Check sheet for the drawn part. Datum: minimum x, y, z corner. Units: mm. A direction names the side the tool comes from. Round coordinates to 2 decimals unless told otherwise and drop trailing zeros. Order: outer loops, then holes, each group sorted by start corner. A loop starts at its lowest first (then second) coordinate and runs counter-clockwise, first axis right, second up. Notation, with made-up numbers: (-15.75, 7) -> (41.25, 7) arc R13 cw to (41.25, 26) -> close; hole circle Ø7 at (-29.75, 34.25). An arc over 180 degrees is marked (long way). Answer as a JSON object with one key per item and string values. Group by question number.
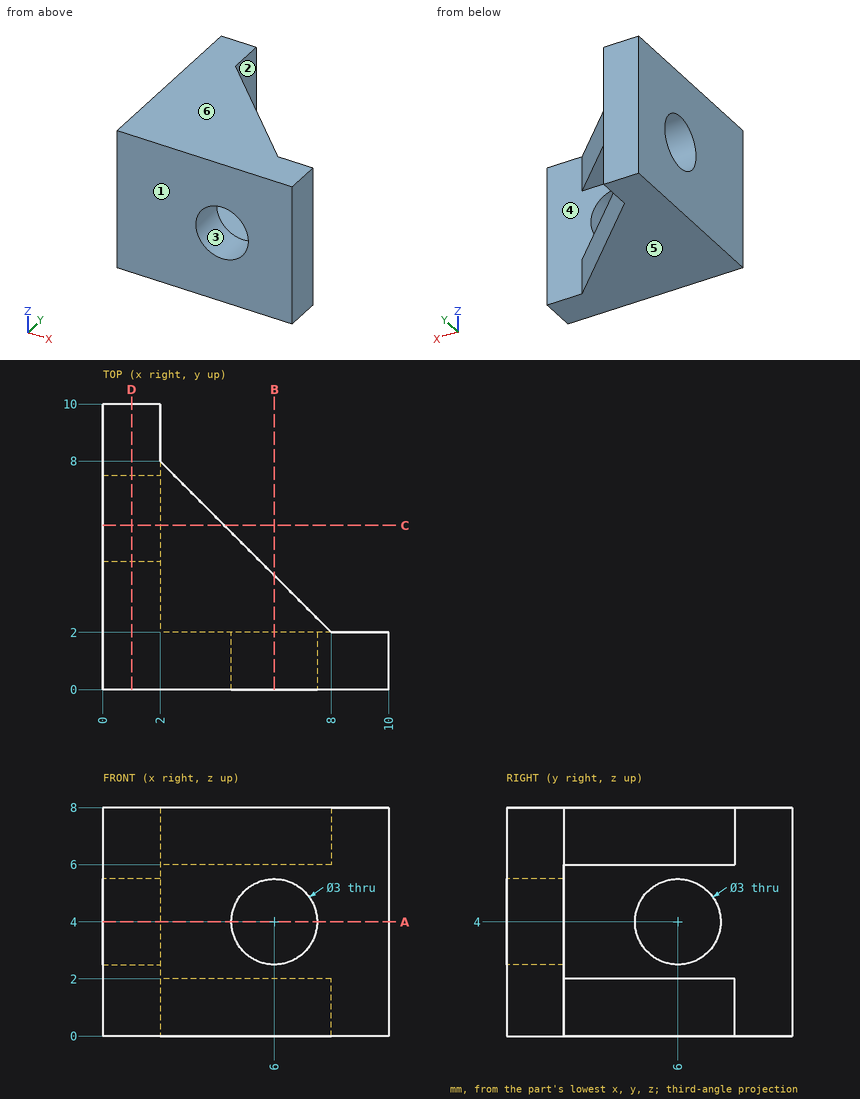
Item 1: Thickness scan on L1, parallel to Z at x = 6, y = 0.5; L2, parallel to Y at x = 0.8, z = 4; L3, parallel to Z at x = 4, y = 2.5. Record the ranges inside material, lowest first.
Item 2: Sectioned sample at D-D, the plane x = 1. Enter the section's corners in (y, z).
Item 3: Sectioned sample at A-A, the plane z = 4. Enter the section's corners in (x, y), then the cut area to 3 significant figures.
Item 4: Mould release check, pull along Z, two halves, no side actions. Record for the marked faces 3, 4, 5 and 6: pulls with the +Z half, pulls with the -Z half, needs draft (parallel to the pull), parting line crosses it, or undercut.
Item 5: Set-up check for the marked faces 1 and 2: record each of +Z, -Z, +X, -X, +Y, -Y from which the full face is reachable in a straight line by a thin tool's end or side.
Item 6: Sectioned sample at B-B, the plane x = 6. Enter the section's corners in (y, z).
Item 7: Depth check by flat-ended pin: pin 1 Ø1 at (y, z) = (3, 2) entering from +X; pin 2 Ø3 at (y, z) = (8.5, 2.5) entering from +X. Enter the tip coordinate at first touch or a pass-through.
Item 8: Sectioned sample at C-C, the plane y = 5.75. Enter the section's corners in (x, z).
Result:
{
 "1": {"L1": "z = 0 to 2.5, 5.5 to 8", "L2": "y = 0 to 4.5, 7.5 to 10", "L3": "z = 0 to 2, 6 to 8"},
 "2": {"outline": "(0, 0) -> (10, 0) -> (10, 8) -> (0, 8) -> close; hole circle Ø3 at (6, 4)"},
 "3": {"outline": "(0, 0) -> (4.5, 0) -> (4.5, 2) -> (2, 2) -> (2, 4.5) -> (0, 4.5) -> close; (0, 7.5) -> (2, 7.5) -> (2, 10) -> (0, 10) -> close; (7.5, 0) -> (10, 0) -> (10, 2) -> (7.5, 2) -> close", "area": "24.0 mm2"},
 "4": {"face 3": "undercut", "face 4": "undercut", "face 5": "pulls with the -Z half", "face 6": "pulls with the +Z half"},
 "5": {"face 1": "+Z, -Z, +X, -X, -Y", "face 2": "+X, +Y"},
 "6": {"outline": "(0, 0) -> (4, 0) -> (4, 2) -> (2, 2) -> (2, 2.5) -> (0, 2.5) -> close; (0, 5.5) -> (2, 5.5) -> (2, 6) -> (4, 6) -> (4, 8) -> (0, 8) -> close"},
 "7": {"pin 1": "stops at x = 7.5", "pin 2": "stops at x = 2.91"},
 "8": {"outline": "(0, 0) -> (4.25, 0) -> (4.25, 2) -> (2, 2) -> (2, 2.52) -> (0, 2.52) -> close; (0, 5.48) -> (2, 5.48) -> (2, 6) -> (4.25, 6) -> (4.25, 8) -> (0, 8) -> close"}
}
